Here's how the part is built. I have some questions about the finished solid (model axes, mm). Face numbers are marked on the shaded views. A direction names the side the tool comes from. Round coordinates to 2 decimals unless told otherwise and drop trailing zeros. Write each loop counter-clockwise with the first axis right and the second up, starting at its lowest first coordinate (ties: lowest second). Pieces come first, ordered by that corner, then holes. Notation, with made-up numbers: (4, 38) -> (11, 38) arc R12 ccw to (11, 50) -> close; hole circle Ø3 at (49.25, -26.75). An arc over 180 degrees is marked (long way). Answer as CSV lines item,"result".
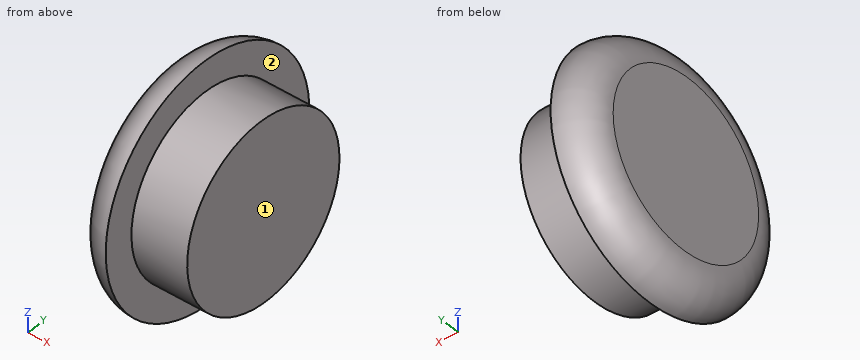
from build123d import *

# Parameters (mm, degrees)
SKETCH1_R           = 7.85
BOSS_EXTRUDE1_DEPTH = 5
SKETCH1_3_R         = 10.5
BOSS_EXTRUDE2_DEPTH = 3
FILLET1_R           = 3


with BuildPart() as part:
    # Sketch1 → Boss-Extrude1 (new body)
    with BuildSketch(Plane(origin=(0, 0, 0), x_dir=(0, 0, -1), z_dir=(1, 0, 0))):
        Circle(SKETCH1_R)
    extrude(amount=BOSS_EXTRUDE1_DEPTH)

    # Sketch1<3> → Boss-Extrude2 (add)
    with BuildSketch(Plane(origin=(0, 0, 0), x_dir=(0, 0, -1), z_dir=(1, 0, 0))):
        Circle(SKETCH1_3_R)
    extrude(amount=-BOSS_EXTRUDE2_DEPTH)

    # Fillet1
    fillet1_edges = [part.edges().sort_by_distance(p)[0] for p in [
        (-3, 0, 10.5),
    ]]
    fillet(fillet1_edges, radius=FILLET1_R - 0.0001)  # a hair under: the kernel refuses the full size


solid = part.part
Item 1: Suppose I cut it at C-C, the plane x = 0.5. List the corners of the cut face in (y, z) for me.
Results found:
outline,"circle Ø15.7 at (0, 0)"
Item 2: For the marked faces 1 and 2, which set-ups out of +Z, -Z, +X, -X, +Y, -Y let a thin tool reach every point of the face, with its end or its side?
Results found:
face 1,"+Z, -Z, +X, +Y, -Y"
face 2,"+X"
Item 3: I need wall thicknesses on L1, parallel to Y at x = 0.5, z = 0.25; L2, parallel to Z at x = 3, y = 4; L3, parallel to Y at x = -1.5, z = 1.25. Which ranges of each line are inside material? Lowest first, please.
Results found:
L1,"y = -7.85 to 7.85"
L2,"z = -6.75 to 6.75"
L3,"y = -10.02 to 10.02"
Item 4: Will these pins go through, and if not, where does the flat tip stop? pin 1 (3 mm diameter, centred on x = 2.5, z = -5.5, fed in from -Y); pin 2 (1 mm diameter, centred on x = 0, y = 3, fed in from -Z); pin 3 (2 mm diameter, centred on x = 2, z = 4.5, fed in from +Y).
Results found:
pin 1,"stops at y = -6.75"
pin 2,"stops at z = -10.2"
pin 3,"stops at y = 7.03"
